```python
from build123d import *

# Parameters (mm, degrees)
RESSALTO_EXTRUS_O1_DEPTH = 4


with BuildPart() as part:
    # Esboço1 → Ressalto-extrusão1 (new body)
    with BuildSketch(Plane.XY):
        with BuildLine():
            Line((0.1, 0), (0.1, 0.8))
            Line((0.1, 0.8), (13.5, 0.8))
            Line((13.5, 0.8), (13.5, 1))
            Line((13.5, 1), (0, 1))
            ThreePointArc((0, 1), (-0.070710678, 0.970710678), (-0.1, 0.9))
            Line((-0.1, 0.9), (-0.1, 0.8))
            Line((-0.1, 0.8), (-0.1, 0))
            ThreePointArc((-0.1, 0), (0, -0.1), (0.1, 0))
        make_face()
    extrude(amount=RESSALTO_EXTRUS_O1_DEPTH)


solid = part.part
```
Could you check a few things on this model? Use its own coordinates, in mm. A direction names the side the tool comes from. Round coordinates to 2 decimals unless told otherwise and drop trailing zeros. Loops run counter-clockwise (first coordinate to the right, second up) from the corner with the lowest first, then second, coordinate; pieces in that order, holes last.
Q1. Please list where these lines run through material, in increasing order: L1, parallel to Y at x = 12.75, z = 3.25; L2, parallel to X at y = 0.7, z = 1.3.
Q2. I want a section at A-A (z = 1.4). Write out the boundary of the cut face in (x, y).
Q3. For P1, Ø1.2, axis at x = 5.5, z = 2, coming from the -Y side, with a flat end and sliding along its axis, tell me the tip position at first contact or that it passes through.
Q4. I want a section at C-C (x = 6.25). Write out the boundary of the cut face in (y, z), and give its area (3 significant figures).
Q5. On a 3-axis mill with a long thin cutter (end or side, diameter ignored), from which of +Z, -Z, +X, -X, +Y, -Y can I reach the whole of each face in a straight line? I mean faces 1 (the flat face through (7, 1, 2)), 2 (the flat face through (7, 0.8, 2)). Say none if no direction works.
Q6. I want a section at B-B (y = 0.15). Write out the boundary of the cut face in (x, z), and give its area (3 significant figures).
Answer below:
1. L1: y = 0.8 to 1
1. L2: x = -0.1 to 0.1
2. outline: (-0.1, 0) arc R0.1 ccw to (0.1, 0) - (0.1, 0.8) - (13.5, 0.8) - (13.5, 1) - (0, 1) arc R0.1 ccw to (-0.1, 0.9) - close
3. P1: stops at y = 0.8
4. outline: (0.8, 0) - (1, 0) - (1, 4) - (0.8, 4) - close
4. area: 0.800 mm2
5. face 1: +Z, -Z, +X, -X, +Y
5. face 2: +Z, -Z, +X, -Y
6. outline: (-0.1, 0) - (0.1, 0) - (0.1, 4) - (-0.1, 4) - close
6. area: 0.800 mm2
